Source: CAD feature listing. Evaluate the final solid. Frame: model axes, mm. Coordinates: 2 decimals unless noted, no trailing zeros. Loops run counter-clockwise (first coordinate to the right, second up) from the corner with the lowest first, then second, coordinate; pieces in that order, holes last.
Item 1: Section query B-B, the plane z = -2.5. Return the cut outline in (x, y).
Item 2: Section query D-D, the plane y = 0.7. State how many separate pieces and enclosed holes the cut face has, then the cut area to 3 significant figures.
Item 3: Pull-direction query (X, two-part tool) for faces 1 (the flat face through (0, 2, -4)), 2 (the cylindrical face through (2.96, 1.55, -6.47)), 3 (the cylindrical face through (4.636, 1.578, -2.285)); classes: +X half, -X half, draft (parallel to the pull), parting line (faces both ways), or undercut.
Item 4: Section query C-C, the plane z = -6.5. Return the cut outline in (x, y), then the cut area to 3 significant figures.
Item 5: Section query A-A, the plane y = 2.35. Return the cut outline in (x, z), then the cut area to 3 significant figures.
Item 6: Line query: probe 1 along X at (y, z) = (2, -2.5); probe 2 along Z at (x, y) = (2.75, 0.35); probe 3 along Z at (x, y) = (3.75, 3.6). Output: solid intervals per line, ascending.
```python
from build123d import *

# Parameters (mm, degrees)
EXTRUDE_1_DEPTH     = 6
SKETCH_2_R          = 1.65
CUT_EXTRUDE_1_DEPTH = 6
FILLET_1_R          = 1
CHAMFER_1_SIZE      = 0.8
FILLET_2_R          = 0.5
FILLET_3_R          = 0.3


with BuildPart() as part:
    # 草圖1 → 填料-伸長1 (new body)
    with BuildSketch(Plane(origin=(0, 0, 0), x_dir=(0, 0, -1), z_dir=(1, 0, 0))):
        with BuildLine():
            Line((0, 0), (4.95, 0))
            ThreePointArc((4.95, 0), (6.5, 1.55), (8.05, 0))
            Line((8.05, 0), (9, 0))
            Line((9, 0), (9, 4))
            Line((9, 4), (0, 4))
            Line((0, 4), (0, 0))
        make_face()
    extrude(amount=EXTRUDE_1_DEPTH)

    # 草圖2 → 除料-伸長1 (cut)
    with BuildSketch(Plane(origin=(0, 0, 0), x_dir=(-1, 0, 0), z_dir=(0, -1, 0))):
        with Locations(Location((-3, 2.5, 0), (0, 0, 90))):
            Circle(SKETCH_2_R)
    extrude(amount=-CUT_EXTRUDE_1_DEPTH, mode=Mode.SUBTRACT)

    # 圓角1
    fillet_1_edges = [part.edges().sort_by_distance(p)[0] for p in [
        (6, 2, -9),
        (6, 2, 0),
        (0, 2, -9),
        (0, 2, 0),
    ]]
    fillet(fillet_1_edges, radius=FILLET_1_R)

    # 導角1
    chamfer_1_edges = [part.edges().sort_by_distance(p)[0] for p in [
        (3, 4, -0.85),
    ]]
    chamfer(chamfer_1_edges, length=CHAMFER_1_SIZE)

    # 圓角2
    # the kernel refuses this fillet: 0.5 mm, written as the material it takes off along each edge
    with BuildSketch(Plane(origin=(6, 4, -8), x_dir=(-1, 0, 0), z_dir=(0, 0, 1))) as fillet_2_piece_1:
        with BuildLine():
            CenterArc((FILLET_2_R, FILLET_2_R), FILLET_2_R, 180, 90)
            Line((0, FILLET_2_R), (0, 0))
            Line((0, 0), (FILLET_2_R, 0))
        make_face()
    extrude(amount=7, mode=Mode.SUBTRACT)
    with BuildSketch(Plane(origin=(0, 4, -8), x_dir=(1, 0, 0), z_dir=(0, 0, 1))) as fillet_2_piece_2:
        with BuildLine():
            CenterArc((FILLET_2_R, -FILLET_2_R), FILLET_2_R, 90, 90)
            Line((0, -FILLET_2_R), (0, 0))
            Line((0, 0), (FILLET_2_R, 0))
        make_face()
    extrude(amount=7, mode=Mode.SUBTRACT)
    with BuildSketch(Plane(origin=(1, 4, 0), x_dir=(0, 0, -1), z_dir=(1, 0, 0))) as fillet_2_piece_3:
        with BuildLine():
            CenterArc((FILLET_2_R, -FILLET_2_R), FILLET_2_R, 90, 90)
            Line((0, -FILLET_2_R), (0, 0))
            Line((0, 0), (FILLET_2_R, 0))
        make_face()
    extrude(amount=4, mode=Mode.SUBTRACT)
    with BuildSketch(Plane(origin=(1, 4, -9), x_dir=(0, 0, 1), z_dir=(1, 0, 0))) as fillet_2_piece_4:
        with BuildLine():
            CenterArc((FILLET_2_R, FILLET_2_R), FILLET_2_R, 180, 90)
            Line((0, FILLET_2_R), (0, 0))
            Line((0, 0), (FILLET_2_R, 0))
        make_face()
    extrude(amount=4, mode=Mode.SUBTRACT)
    with BuildSketch(Plane(origin=(1, 4, -1), x_dir=(0, 0, 1), z_dir=(1, 0, 0))) as fillet_2_piece_5:
        with BuildLine():
            CenterArc((1 - FILLET_2_R, FILLET_2_R), FILLET_2_R, 270, 90)
            Line((1, FILLET_2_R), (1, 0))
            Line((1, 0), (1 - FILLET_2_R, 0))
        make_face()
    revolve(axis=Axis((1, 4, -1), (0, -1, 0)), revolution_arc=90, mode=Mode.SUBTRACT)
    with BuildSketch(Plane(origin=(5, 4, -1), x_dir=(0, 0, 1), z_dir=(-1, 0, 0))) as fillet_2_piece_6:
        with BuildLine():
            CenterArc((1 - FILLET_2_R, -FILLET_2_R), FILLET_2_R, 0, 90)
            Line((1, -FILLET_2_R), (1, 0))
            Line((1, 0), (1 - FILLET_2_R, 0))
        make_face()
    revolve(axis=Axis((5, 4, -1), (0, 1, 0)), revolution_arc=90, mode=Mode.SUBTRACT)
    with BuildSketch(Plane(origin=(1, 4, -8), x_dir=(-1, 0, 0), z_dir=(0, 0, 1))) as fillet_2_piece_7:
        with BuildLine():
            CenterArc((1 - FILLET_2_R, FILLET_2_R), FILLET_2_R, 270, 90)
            Line((1, FILLET_2_R), (1, 0))
            Line((1, 0), (1 - FILLET_2_R, 0))
        make_face()
    revolve(axis=Axis((1, 4, -8), (0, -1, 0)), revolution_arc=90, mode=Mode.SUBTRACT)
    with BuildSketch(Plane(origin=(5, 4, -8), x_dir=(1, 0, 0), z_dir=(0, 0, 1))) as fillet_2_piece_8:
        with BuildLine():
            CenterArc((1 - FILLET_2_R, -FILLET_2_R), FILLET_2_R, 0, 90)
            Line((1, -FILLET_2_R), (1, 0))
            Line((1, 0), (1 - FILLET_2_R, 0))
        make_face()
    revolve(axis=Axis((5, 4, -8), (0, 1, 0)), revolution_arc=90, mode=Mode.SUBTRACT)

    # 圓角3
    fillet_3_edges = [part.edges().sort_by_distance(p)[0] for p in [
        (6, 1.537449186, -6.303149803),
        (0.000701488, 0.196850436, -8.037449158),
        (5.999298512, 0.196850436, -8.037449158),
        (0, 1.537449186, -6.303149803),
    ]]
    fillet(fillet_3_edges, radius=FILLET_3_R)


solid = part.part
```
Verdict:
1. outline: (0, 0) - (1.35, 0) - (1.35, 3.2) - (0.55, 4) - (0.5, 4) arc R0.5 ccw to (0, 3.5) - close; (4.65, 0) - (6, 0) - (6, 3.5) arc R0.5 ccw to (5.5, 4) - (5.45, 4) - (4.65, 3.2) - close
2. separate pieces: 2
2. enclosed holes: 1
2. area: 27.9 mm2
3. face 1: -X half
3. face 2: draft
3. face 3: undercut
4. outline: (0, 1.85) arc R0.3 ccw to (0.3, 1.55) - (5.7, 1.55) arc R0.3 ccw to (6, 1.85) - (6, 3.5) arc R0.5 ccw to (5.5, 4) - (0.5, 4) arc R0.5 ccw to (0, 3.5) - close
4. area: 14.6 mm2
5. outline: (0, -8) arc R1 ccw to (1, -9) - (5, -9) arc R1 ccw to (6, -8) - (6, -1) arc R1 ccw to (5, 0) - (1, 0) arc R1 ccw to (0, -1) - close; hole circle Ø3.3 at (3, -2.5)
5. area: 44.6 mm2
6. probe 1: x = 0 to 1.35, 4.65 to 6
6. probe 2: z = -9 to -8.01, -4.99 to -4.13, -0.87 to 0
6. probe 3: z = -8.99 to -4.41, -0.59 to -0.01
